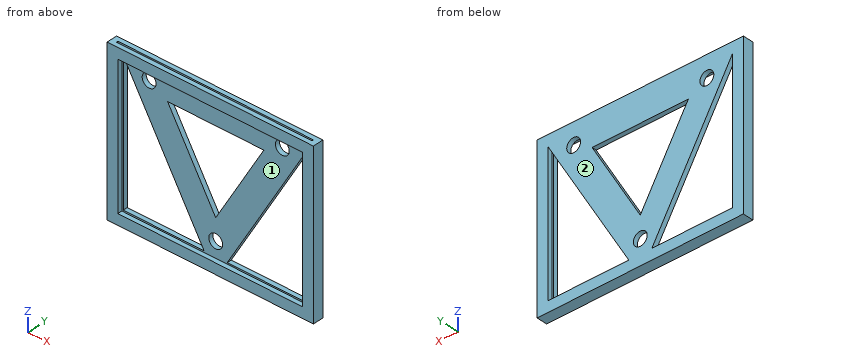
from build123d import *

# Parameters (mm, degrees)
SKETCH1_R           = 6.5
BOSS_EXTRUDE1_DEPTH = 5
SKETCH1_8_W         = 193.5
SKETCH1_8_H         = 151.5
SKETCH1_8_W_2       = 173.5
SKETCH1_8_H_2       = 131.5
BOSS_EXTRUDE2_DEPTH = 5
SKETCH2_W           = 183.5
SKETCH2_H           = 146.5
CUT_EXTRUDE2_DEPTH  = 0.75


with BuildPart() as part:
    # Sketch1 → Boss-Extrude1 (new body)
    with BuildSketch(Plane(origin=(0, 0, 0), x_dir=(1, 0, 0), z_dir=(0, 1, 0))):
        Polygon((10.828439602, 85.415608176), (-10.828439602, 85.415608176), (-86.75, -46.084391824), (86.75, -46.084391824), align=None)
        with Locations(Location((-62.5, -36.084391824, 0), (0, 0, 270))):
            Circle(SKETCH1_R, mode=Mode.SUBTRACT)
        with Locations(Location((62.5, -36.084391824, 0), (0, 0, 270))):
            Circle(SKETCH1_R, mode=Mode.SUBTRACT)
        Polygon((-45.179491924, -26.084391824), (0, 52.168783649), (45.179491924, -26.084391824), align=None, mode=Mode.SUBTRACT)
        with Locations(Location((0, 72.168783649, 0), (0, 0, 270))):
            Circle(SKETCH1_R, mode=Mode.SUBTRACT)
    extrude(amount=BOSS_EXTRUDE1_DEPTH)

    # Sketch1_8 → Boss-Extrude2 (add, symmetric)
    with BuildSketch(Plane(origin=(0, 0, 0), x_dir=(1, 0, 0), z_dir=(0, 1, 0))):
        with Locations((0, 19.665608176)):
            Rectangle(SKETCH1_8_W, SKETCH1_8_H)
        with Locations((0, 19.665608176)):
            Rectangle(SKETCH1_8_W_2, SKETCH1_8_H_2, mode=Mode.SUBTRACT)
    extrude(amount=BOSS_EXTRUDE2_DEPTH, both=True)

    # Sketch2 → Cut-Extrude2 (cut, symmetric)
    with BuildSketch(Plane(origin=(0, 0, 0), x_dir=(1, 0, 0), z_dir=(0, 1, 0))):
        with Locations((0, 17.165608176)):
            Rectangle(SKETCH2_W, SKETCH2_H)
    extrude(amount=CUT_EXTRUDE2_DEPTH, both=True, mode=Mode.SUBTRACT)


solid = part.part
Input: part model. Units: mm. Frame: model coordinates. Face numbers are marked on the shaded views. Give positions to 0.01 mm unless a question says otherwise; leave off trailing zeros. Write each loop counter-clockwise with the first axis right and the second up, starting at its lowest first coordinate (ties: lowest second). Pieces come first, ordered by that corner, then holes. Notation, with made-up numbers: M 84.5,-32.5 L 89.5,-32.5 A13 ccw 89.5,-21.5 Z; hole C -11.5,-4 d8. An arc over 180 degrees is marked long. Use one line per item in the form item = value.
1. Cut plane C-C on z = -24. Return loops of the section in (x, y).
Outcome:
outline = M -96.75,-5 L -86.75,-5 L -86.75,-0.75 L -91.75,-0.75 L -91.75,0.75 L -86.75,0.75 L -86.75,5 L -96.75,5 Z; M -46.29,0.75 L -16.26,0.75 L -16.26,5 L -46.29,5 Z; M 16.26,0.75 L 46.29,0.75 L 46.29,5 L 16.26,5 Z; M 86.75,-5 L 96.75,-5 L 96.75,5 L 86.75,5 L 86.75,0.75 L 91.75,0.75 L 91.75,-0.75 L 86.75,-0.75 Z
2. Cut plane B-B on y = 3.5. Return loops of the section in (x, z), and give its area (3 significant figures).
Outcome:
outline = M -96.75,-95.42 L 96.75,-95.42 L 96.75,56.08 L -96.75,56.08 Z; hole M -86.75,-85.42 L -10.83,-85.42 L -86.75,46.08 Z; hole C -62.5,36.08 d13; hole M -45.18,26.08 L 0,-52.17 L 45.18,26.08 Z; hole C 0,-72.17 d13; hole M 10.83,-85.42 L 86.75,-85.42 L 86.75,46.08 Z; hole C 62.5,36.08 d13
area = 15,400 mm²
3. Cut plane A-A on z = -63. Return loops of the section in (x, y).
Outcome:
outline = M -96.75,-5 L -86.75,-5 L -86.75,-0.75 L -91.75,-0.75 L -91.75,0.75 L -86.75,0.75 L -86.75,5 L -96.75,5 Z; M -23.77,0.75 L 23.77,0.75 L 23.77,5 L -23.77,5 Z; M 86.75,-5 L 96.75,-5 L 96.75,5 L 86.75,5 L 86.75,0.75 L 91.75,0.75 L 91.75,-0.75 L 86.75,-0.75 Z
4. First-contact query: P1, Ø15, axis at x = 62.5, z = 36.08, coming from the -Y side. Flat tip, straight axial feed; report the tip coordinate or a pass-through.
Outcome:
P1 = 0.75
5. Cut plane D-D on x = -62.5. Return loops of the section in (y, z).
Outcome:
outline = M -5,-95.42 L 5,-95.42 L 5,-85.42 L 0.75,-85.42 L 0.75,-90.42 L -0.75,-90.42 L -0.75,-85.42 L -5,-85.42 Z; M -5,46.08 L -0.75,46.08 L -0.75,56.08 L -5,56.08 Z; M 0.75,4.08 L 5,4.08 L 5,29.58 L 0.75,29.58 Z; M 0.75,42.58 L 5,42.58 L 5,56.08 L 0.75,56.08 Z
6. Mould query, pull axis X, two halves, no side actions, for the marked faces 1 and 2. Classes: released by +X, released by -X, zero draft, split by the parting line, or undercut.
Outcome:
face_1 = undercut
face_2 = zero draft
7. Ray query, L1, parallel to Z at x = 0, y = 3.9; L2, parallel to Z at x = 62.5, y = 3.9; L3, parallel to Z at x = 62, y = -2.5. Return the intervals inside material, ascending.
Outcome:
L1 = -95.42 to -78.67, -65.67 to -52.17, 26.08 to 56.08
L2 = -95.42 to -85.42, 4.08 to 29.58, 42.58 to 56.08
L3 = -95.42 to -85.42, 46.08 to 56.08
